Input: part model. Units: mm. Frame: model coordinates. A direction names the side the tool comes from. Give positions to 0.01 mm unless a question says otherwise; leave off trailing zeros. Loops run counter-clockwise (first coordinate to the right, second up) from the corner with the lowest first, then second, coordinate; pieces in that order, holes last. Notation, with made-up numbers: (46, -33) -> (54, -33) arc R29 ccw to (54, -4) -> close; hole circle Ø3 at (-22.75, 5). An arc over 180 degrees is marked (long way). Answer as a JSON object with one key per item and string values.
Autodesk Inventor part; units mm, degrees
ref_plane "YZ Plane" through (0, 0, 0) normal (1, 0, 0) x (0, 1, 0)
ref_plane "XZ Plane" through (0, 0, 0) normal (0, 1, 0) x (-1, 0, 0)
ref_plane "XY Plane" through (0, 0, 0) normal (0, 0, 1) x (1, 0, 0)
sketch "Sketch1" plane through (0, 0, 0) normal (0, 0, 1) x (1, 0, 0)
  line L0 (0, 0) -> (50.8, 0)
  line L1 (50.8, 0) -> (50.8, 50.8)
  line L2 (50.8, 50.8) -> (0, 50.8)
  line L3 (0, 50.8) -> (0, 0)
  line L4 (0, 0) -> (4.7625, 0) construction
  line L5 (4.7625, 0) -> (4.7625, 4.7625) construction
  line L6 (4.7625, 4.7625) -> (0, 4.7625) construction
  line L7 (0, 4.7625) -> (0, 0) construction
  line L8 (50.8, 50.8) -> (46.0375, 50.8) construction
  line L9 (46.0375, 50.8) -> (46.0375, 46.0375) construction
  line L10 (46.0375, 46.0375) -> (50.8, 46.0375) construction
  line L11 (50.8, 46.0375) -> (50.8, 50.8) construction
  line L12 (46.0375, 46.0375) -> (4.7625, 46.0375)
  line L13 (4.7625, 46.0375) -> (4.7625, 4.7625)
  line L14 (4.7625, 4.7625) -> (46.0375, 4.7625)
  line L15 (46.0375, 4.7625) -> (46.0375, 46.0375)
  dimension "d0" = 50.8
  dimension "d1" = 50.8
  dimension "d2" = 4.7625
  dimension "d3" = 4.7625
  dimension "d4" = 4.7625
  dimension "d5" = 4.7625
extrude "Extrusion1" add sketch "Sketch1" along normal blind 812.8
sketch "Sketch2" plane through (50.8, 0, 0) normal (1, 0, 0) x (0, 0, -1)
  line L0 (0, 4.7625) -> (-812.8, 4.7625)
  line L1 (0, 46.0375) -> (-812.8, 46.0375)
  line L2 (0, 4.7625) -> (-63.5, 4.7625)
  line L3 (-63.5, 4.7625) -> (-63.5, 46.0375)
  line L4 (-63.5, 46.0375) -> (0, 46.0375)
  line L5 (0, 46.0375) -> (0, 4.7625)
  line L6 (-812.8, 4.7625) -> (-812.8, 46.0375)
  line L7 (-812.8, 4.7625) -> (-749.3, 4.7625)
  line L8 (-749.3, 4.7625) -> (-749.3, 46.0375)
  line L9 (-749.3, 46.0375) -> (-812.8, 46.0375)
  line L10 (-812.8, 46.0375) -> (-812.8, 4.7625)
  point P0 (0, 0)
  dimension "d8" = 63.5
  dimension "d9" = 63.5
extrude "Extrusion2" cut sketch "Sketch2" against normal blind 50.8 contours L0 L3 L1 L5 | L0 L6 L1 L8
sketch "Sketch3" plane through (0, 0, 0) normal (0, -1, 0) x (1, 0, 0)
  line L0 (46.0375, 63.5) -> (46.0375, 749.3)
  line L1 (4.7625, 63.5) -> (0, 63.5)
  line L2 (46.0375, 63.5) -> (4.7625, 63.5)
  line L3 (25.4, 63.5) -> (25.4, 0)
  line L4 (50.8, 749.3) -> (46.0375, 749.3)
  line L5 (4.7625, 749.3) -> (0, 749.3)
  line L6 (46.0375, 749.3) -> (4.7625, 749.3)
  line L7 (25.4, 749.3) -> (25.4, 812.8)
  line L8 (0, 812.8) -> (50.8, 812.8)
  point P0 (0, 0)
  point P1 (25.4, 31.75)
  point P2 (25.4, 781.05)
hole "Hole1" at (25.4, 0, 31.75) at (25.4, 0, 781.05) direction (0, 1, 0) diameter 9.525 depth 50.8 tip angle 118
equation "\"d0\" = d1"
equation "\"d2\" = d3"
equation "\"d4\" = d3"
equation "\"d5\" = d3"
properties part number "32in2.0Sq" material "Steel, Mild"
Q1. Section C-C, the plane x = 37.5. Return the cut outline in (y, z).
Evaluation:
{"outline": "(0, 0) -> (4.76, 0) -> (4.76, 812.8) -> (0, 812.8) -> close; (46.04, 0) -> (50.8, 0) -> (50.8, 812.8) -> (46.04, 812.8) -> close"}
Q2. Draft query along Y for faces 3 (the flat face through (50.8, 25, 401)), 4 (the flat face through (46.038, 25, 402)), 5 (the flat face through (26, 4.762, 401)), 6 (the flat face through (25, 0, 401)). Return one class per face: +Y half, -Y half, draft (parallel to the pull), parting line (faces both ways), or undercut.
Evaluation:
{"face 3": "draft", "face 4": "undercut", "face 5": "undercut", "face 6": "-Y half"}
Q3. Ray query, line 1 along Z through (x, y) = (25.4, 1.05); line 2 along X through (y, z) = (49.4, 31.75); line 3 along X through (y, z) = (11, 201.5). Return the intervals inside material, ascending.
Evaluation:
{"line 1": "z = 0 to 26.99, 36.51 to 776.29, 785.81 to 812.8", "line 2": "x = 0 to 20.64, 30.16 to 50.8", "line 3": "x = 0 to 4.76, 46.04 to 50.8"}
Q4. Access query for faces 1 (the flat face through (0, 26, 401)), 2 (the flat face through (4.762, 26, 402)). Directions: +Z, -Z, +X, -X, +Y, -Y. A direction counts if a zero-diameter tool reaches every point of the face in a straight line with its end or side. Return the directions, or none.
Evaluation:
{"face 1": "+Z, -Z, -X, +Y, -Y", "face 2": "+Z, -Z"}
Q5. Section B-B, the plane z = 349.5. Return the cut outline in (x, y).
Evaluation:
{"outline": "(0, 0) -> (50.8, 0) -> (50.8, 50.8) -> (0, 50.8) -> close; hole (4.76, 4.76) -> (46.04, 4.76) -> (46.04, 46.04) -> (4.76, 46.04) -> close"}
Q6. Pin query (flat end, axial travel): pin 1 (2.5 mm diameter, centred on x = 49.5, y = 26, fed in from -Z); pin 2 (7.5 mm diameter, centred on x = 25.4, z = 781.05, fed in from -Y); pin 3 (5 mm diameter, centred on x = 1.5, y = 19, fed in from +Z). Return the tip coordinate at first contact, or that it passes through.
Evaluation:
{"pin 1": "stops at z = 63.5", "pin 2": "passes through", "pin 3": "stops at z = 749.3"}
Q7. Section A-A, the plane y = 25.5. Return the cut outline in (x, z).
Evaluation:
{"outline": "(0, 63.5) -> (4.76, 63.5) -> (4.76, 749.3) -> (0, 749.3) -> close; (46.04, 63.5) -> (50.8, 63.5) -> (50.8, 749.3) -> (46.04, 749.3) -> close"}
